Can you work these out from the model? Positions are in its coordinate system, mm. A direction names the side the tool comes from. Give positions to 0.01 mm unless a question says otherwise; leave off trailing zeros. Order: outer loops, then holes, each group sorted by start corner. A loop starts at its lowest first (then second) coordinate and runs counter-clockwise, first axis right, second up. Notation, with made-up numbers: (-10.5, 3.5) -> (25.5, 3.5) arc R19 cw to (25.5, 20.5) -> close; hole circle Ø6 at (-26.75, 70). An arc over 180 degrees is marked (long way). Answer as CSV lines item,"result".
Autodesk Inventor part; units mm, degrees
ref_plane "YZ Plane" through (0, 0, 0) normal (1, 0, 0) x (0, 1, 0)
ref_plane "XZ Plane" through (0, 0, 0) normal (0, 1, 0) x (-1, 0, 0)
ref_plane "XY Plane" through (0, 0, 0) normal (0, 0, 1) x (1, 0, 0)
sketch "Sketch1" plane through (0, 0, 0) normal (0, 0, 1) x (1, 0, 0)
  circle A0 centre (0, 0) radius 5.5
  circle A1 centre (0, 0) radius 10
  dimension "d0" = 11
  dimension "d1" = 20
extrude "Extrusion1" add sketch "Sketch1" along normal blind 18
sketch "Sketch3" plane through (0, 0, 0) normal (0, 0, -1) x (-1, 0, 0)
  line L0 (15, -15) -> (-15, -15)
  line L1 (-15, -15) -> (-15, 15)
  line L2 (-15, 15) -> (15, 15)
  line L3 (15, 15) -> (15, -15)
  line L4 (15, -15) -> (-15, 15) construction
  line L5 (-15, -15) -> (15, 15) construction
  point P0 (0, 0)
  dimension "d4" = 30
  dimension "d5" = 30
extrude "Extrusion2" add sketch "Sketch3" along normal blind 4
sketch "Sketch5" plane through (0, 0, 0) normal (0, 0, 1) x (1, 0, 0)
  line L0 (-3, 3) -> (3, 3)
  line L1 (3, 3) -> (3, -3)
  line L2 (3, -3) -> (-3, -3)
  line L3 (-3, -3) -> (-3, 3)
  line L4 (-3, 3) -> (3, -3) construction
  line L5 (3, 3) -> (-3, -3) construction
  point P0 (0, 0)
  dimension "d8" = 6
  dimension "d9" = 6
extrude "Extrusion3" cut sketch "Sketch5" against normal blind 10
sketch "Sketch6" plane through (0, 0, 18) normal (0, 0, 1) x (1, 0, 0)
  circle A0 centre (0, 0) radius 10
  line L0 (-10, 0) -> (-5.5, 0) construction
  circle A1 centre (0, 0) radius 5.5
  circle A2 centre (-7.75, 0) radius 1.244
properties part number "MotorDemoV1"
Item 1: Imagine slicing it at D-D, the plane y = 11.25. Please give me the cut outline in (x, z).
Numbers:
outline,"(-15, -4) -> (15, -4) -> (15, 0) -> (-15, 0) -> close"
Item 2: For faces 1 (the flat face through (0, -15, -2)), 2 (the cylindrical face through (-1.19, 5.37, 8.87)), 3 (the flat face through (0, -3, -2)), which set-ups out of +Z, -Z, +X, -X, +Y, -Y let a thin tool reach every point of the face, with its end or its side?
Numbers:
face 1,"+Z, -Z, +X, -X, -Y"
face 2,"+Z"
face 3,"+Z, -Z"
Item 3: Imagine slicing it at A-A, the plane y = 0. Please give me the cut outline in (x, z), then the cut area to 3 significant figures.
Numbers:
outline,"(-15, -4) -> (-3, -4) -> (-3, 0) -> (-5.5, 0) -> (-5.5, 18) -> (-10, 18) -> (-10, 0) -> (-15, 0) -> close; (3, -4) -> (15, -4) -> (15, 0) -> (10, 0) -> (10, 18) -> (5.5, 18) -> (5.5, 0) -> (3, 0) -> close"
area,"258 mm²"
Item 4: Please list where these lines run through material, in increasing order: line 1 along Y through (x, z) = (0, 9.5); line 2 along Z through (x, y) = (6, -13); line 3 along Y through (x, z) = (2.5, 15.75).
Numbers:
line 1,"y = -10 to -5.5, 5.5 to 10"
line 2,"z = -4 to 0"
line 3,"y = -9.68 to -4.9, 4.9 to 9.68"
Item 5: For pin 1 (8 mm diameter, centred on x = -10, y = 10.5, fed in from +Z); pin 2 (1.5 mm diameter, centred on x = 5.5, z = 10.5, fed in from -Y); pin 3 (4 mm diameter, centred on y = -7, z = 1.5, fed in from +X); pin 4 (1.5 mm diameter, centred on y = 8.5, z = 4, fed in from +X), each with a flat end and sliding along its axis, tell me the tip position at first contact or that it passes through.
Numbers:
pin 1,"stops at z = 0"
pin 2,"stops at y = -8.8"
pin 3,"stops at x = 15"
pin 4,"stops at x = 6.32"
Item 6: We'd pull the mould along Y, two halves only. Please class faces 4 (the flat face through (4, -4, 18)), 5 (the flat face through (0, 15, -2)), 6 (the flat face through (-4, 0, 0)): released by +Y, released by -Y, zero draft, split by the parting line, or undercut.
Numbers:
face 4,"zero draft"
face 5,"released by +Y"
face 6,"undercut"
Item 7: Imagine slicing it at C-C, the plane z = 11.75. Please give me the cut outline in (x, y), then the cut area to 3 significant figures.
Numbers:
outline,"circle Ø20 at (0, 0); hole circle Ø11 at (0, 0)"
area,"219 mm²"
